CAD build for the part. Positions are in the model's coordinates, mm. Face numbers are marked on the shaded views. Round coordinates to 2 decimals unless told otherwise and drop trailing zeros. Loops run counter-clockwise (first coordinate to the right, second up) from the corner with the lowest first, then second, coordinate; pieces in that order, holes last.
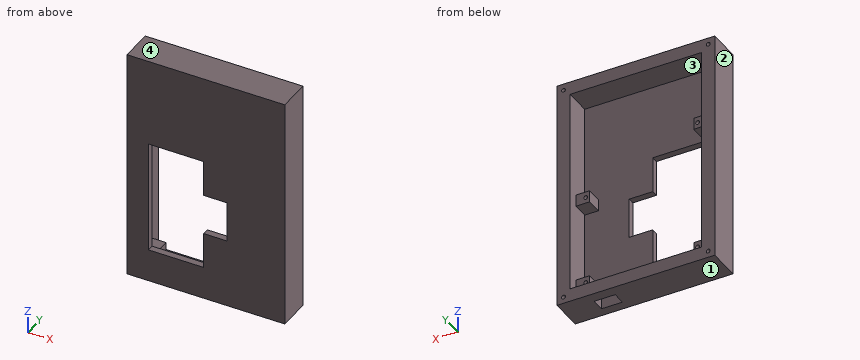
Autodesk Inventor part; units mm, degrees
ref_plane "YZ Plane" through (0, 0, 0) normal (1, 0, 0) x (0, 1, 0)
ref_plane "XZ Plane" through (0, 0, 0) normal (0, 1, 0) x (-1, 0, 0)
ref_plane "XY Plane" through (0, 0, 0) normal (0, 0, 1) x (1, 0, 0)
sketch "Sketch1" plane through (0, 0, 0) normal (0, 1, 0) x (-1, 0, 0)
  line L0 (3.609, 163.5234) -> (-116.891, 163.5234)
  line L1 (-116.891, 163.5234) -> (-116.891, -14.4766)
  line L2 (-116.891, -14.4766) -> (3.609, -14.4766)
  line L3 (3.609, -14.4766) -> (3.609, 163.5234)
  dimension "d1" = 178
  dimension "d2" = 120.5
extrude "Extrusion1" add sketch "Sketch1" along normal blind 25
sketch "Sketch2" plane through (0, 25, 0) normal (0, 1, 0) x (1, 0, 0)
  line L0 (6.391, -153.5234) -> (106.891, -153.5234)
  line L1 (106.891, -153.5234) -> (106.891, 4.4766)
  line L2 (106.891, 4.4766) -> (6.391, 4.4766)
  line L3 (6.391, 4.4766) -> (6.391, -153.5234)
  line L4 (-3.609, -163.5234) -> (116.891, -163.5234)
  line L5 (116.891, -163.5234) -> (116.891, 14.4766)
  point P0 (0, 0)
  dimension "d5" = 158
  dimension "d6" = 100.5
  dimension "d7" = 10
  dimension "d8" = 10
extrude "Extrusion2" cut sketch "Sketch2" against normal blind 20
sketch "Sketch3" plane through (0, 5, 0) normal (0, 1, 0) x (1, 0, 0)
  line L0 (12.891, -96.5234) -> (54.891, -96.5234)
  line L1 (54.891, -96.5234) -> (54.891, -10.5234)
  line L2 (54.891, -10.5234) -> (12.891, -10.5234)
  line L3 (12.891, -10.5234) -> (12.891, -96.5234)
  line L4 (106.891, -153.5234) -> (6.391, -153.5234)
  line L5 (6.391, 4.4766) -> (106.891, 4.4766)
  line L6 (6.391, -153.5234) -> (6.391, 4.4766)
  line L7 (54.891, -69.0234) -> (72.891, -69.0234)
  line L8 (72.891, -69.0234) -> (72.891, -38.0234)
  line L9 (72.891, -38.0234) -> (54.891, -38.0234)
  line L10 (54.891, -38.0234) -> (54.891, -69.0234)
  line L11 (106.891, 4.4766) -> (106.891, -153.5234)
  line L12 (12.891, -55.0234) -> (106.891, -55.0234)
  point P0 (0, 0)
  dimension "d11" = 57
  dimension "d12" = 15
  dimension "d13" = 6.5
  dimension "d14" = 0
  dimension "d15" = 42
  dimension "d16" = 34
  dimension "d17" = 42.5
  dimension "d18" = 84.5
  dimension "d19" = 41.5
  dimension "d20" = 44.5
  dimension "d21" = 14
extrude "Extrusion3" cut sketch "Sketch3" against normal through all contours L3 L12 L1 L0 | L3 L2 L1 L12 | L1 L12 L8 L7 | L1 L9 L8 L12
sketch "Sketch4" plane through (0, 5, 0) normal (0, 1, 0) x (1, 0, 0)
  line L0 (6.391, -7.5234) -> (16.891, -7.5234)
  line L1 (16.891, -7.5234) -> (16.891, 1.4766)
  line L2 (16.891, 1.4766) -> (6.391, 1.4766)
  line L3 (6.391, 1.4766) -> (6.391, -7.5234)
  line L4 (6.391, -153.5234) -> (6.391, 4.4766)
  line L5 (6.391, 4.4766) -> (106.891, 4.4766)
  line L6 (6.391, -153.5234) -> (6.391, 4.4766)
  line L7 (6.391, -53.5234) -> (106.891, -53.5234)
  line L8 (12.891, -10.5234) -> (54.891, -10.5234)
  line L9 (6.391, -99.5234) -> (16.891, -99.5234)
  line L10 (16.891, -99.5234) -> (16.891, -108.5234)
  line L11 (16.891, -108.5234) -> (6.391, -108.5234)
  line L12 (6.391, -108.5234) -> (6.391, -99.5234)
  line L13 (106.891, -153.5234) -> (6.391, -153.5234)
  line L14 (56.641, -153.5234) -> (56.641, 4.4766)
  line L15 (6.391, 4.4766) -> (106.891, 4.4766)
  line L16 (-3.609, 14.4766) -> (-3.609, -163.5234)
  line L17 (106.891, -7.5234) -> (96.391, -7.5234)
  line L18 (96.391, -7.5234) -> (96.391, 1.4766)
  line L19 (96.391, 1.4766) -> (106.891, 1.4766)
  line L20 (106.891, 1.4766) -> (106.891, -7.5234)
  line L21 (108.391, -37.5234) -> (6.391, -37.5234)
  line L22 (106.891, -67.5234) -> (96.391, -67.5234)
  line L23 (106.891, -76.5234) -> (106.891, -67.5234)
  line L24 (96.391, -67.5234) -> (96.391, -76.5234)
  line L25 (96.391, -76.5234) -> (106.891, -76.5234)
  line L26 (54.891, -96.5234) -> (12.891, -96.5234)
  point P0 (0, 0)
  dimension "d24" = 0
  dimension "d25" = 10.5
  dimension "d26" = 9
  dimension "d27" = 3
  dimension "d28" = 43
  dimension "d29" = 60.25
  dimension "d30" = 30
  dimension "d37" = 43
extrude "Extrusion4" add sketch "Sketch4" along normal blind 12 contours L3 L2 L1 L0 | L9 L10 L11 L4 | L17 L18 L19 L20 | L23 L25 L24 L22
sketch "Sketch6" plane through (0, 17, 0) normal (0, 1, 0) x (1, 0, 0)
  circle A0 centre (13.891, -3.0234) radius 1.5
  line L0 (6.391, -153.5234) -> (6.391, 4.4766)
  line L1 (16.891, 1.4766) -> (6.391, 1.4766)
  line L2 (6.391, -53.5234) -> (108.8142, -53.5234)
  line L3 (12.891, -10.5234) -> (54.891, -10.5234)
  line L4 (6.391, -108.5234) -> (16.891, -108.5234)
  circle A1 centre (13.891, -104.0234) radius 1.5
  line L5 (56.641, -153.5234) -> (56.641, 4.4766)
  line L6 (-3.609, 14.4766) -> (-3.609, -163.5234)
  circle A2 centre (99.391, -3.0234) radius 1.5
  line L7 (106.891, -7.5234) -> (106.891, -67.5234)
  line L8 (106.891, -37.5234) -> (6.391, -37.5234)
  line L9 (96.391, -7.5234) -> (106.891, -7.5234)
  circle A3 centre (99.391, -72.0234) radius 1.5
  line L10 (106.891, 4.4766) -> (106.891, -153.5234)
  line L11 (106.891, 1.4766) -> (96.391, 1.4766)
  point P0 (0, 0)
  dimension "d33" = 3
  dimension "d34" = 7.5
  dimension "d35" = 4.5
  dimension "d36" = 43
  dimension "d38" = 110
  dimension "d39" = 4.5
  dimension "d40" = 7.5
  dimension "d41" = 60.25
  dimension "d42" = 30
  dimension "d43" = 69
  dimension "d44" = 7.5
  dimension "d45" = 7.5
  dimension "d46" = 4.5
hole "Hole1" at (13.891, 17, 3.0234) at (13.891, 17, 104.0234) at (99.391, 17, 72.0234) at (99.391, 17, 3.0234) direction (0, -1, 0) diameter 3 depth 10 tip angle 118
thread "Thread1"
thread "Thread2"
thread "Thread3"
thread "Thread4"
sketch "Sketch7" plane through (0, 25, 0) normal (0, 1, 0) x (1, 0, 0)
  circle A0 centre (1.391, -158.5234) radius 1.5
  line L0 (-3.609, -163.5234) -> (116.891, -163.5234)
  line L1 (-3.609, 14.4766) -> (-3.609, -163.5234)
  line L2 (-3.609, 14.4766) -> (-3.609, -163.5234)
  line L3 (-3.609, -74.5234) -> (116.891, -74.5234)
  line L4 (116.891, -163.5234) -> (116.891, 14.4766)
  circle A1 centre (1.391, 9.4766) radius 1.5
  line L5 (56.641, -163.5234) -> (56.641, 14.4766)
  line L6 (116.891, 14.4766) -> (-3.609, 14.4766)
  circle A2 centre (111.891, -158.5234) radius 1.5
  circle A3 centre (111.891, 9.4766) radius 1.5
  point P0 (0, 0)
  dimension "d62" = 3
  dimension "d63" = 5
  dimension "d64" = 5
  dimension "d65" = 89
  dimension "d66" = 60.25
hole "Hole2" at (1.391, 25, 158.5234) at (1.391, 25, -9.4766) at (111.891, 25, -9.4766) at (111.891, 25, 158.5234) direction (0, -1, 0) diameter 3 depth 20 tip angle 118
thread "Thread5"
thread "Thread6"
thread "Thread7"
thread "Thread8"
sketch "Sketch8" plane through (6.391, 25, -4.4766) normal (0, 0, 1) x (1, 0, 0)
  line L0 (70.5, -18) -> (86.5, -18)
  line L1 (86.5, -18) -> (86.5, -8)
  line L2 (86.5, -8) -> (70.5, -8)
  line L3 (70.5, -8) -> (70.5, -18)
  line L4 (100.5, 0) -> (100.5, -20)
  line L5 (0, 0) -> (100.5, 0)
  line L6 (0, -20) -> (100.5, -20)
  point P0 (-6.391, -25)
  dimension "d82" = 14
  dimension "d83" = 16
  dimension "d84" = 8
  dimension "d85" = 2
extrude "Extrusion5" cut sketch "Sketch8" against normal through all
properties part number "cabin_front"
Item 1: Cut at C-C, the plane y = 22. Give the cut face in (x, z).
Answers follow:
outline: (-3.61, -14.48) - (116.89, -14.48) - (116.89, 163.52) - (-3.61, 163.52) - close; hole circle Ø3 at (1.39, -9.48); hole circle Ø3 at (1.39, 158.52); hole (6.39, -4.48) - (106.89, -4.48) - (106.89, 153.52) - (6.39, 153.52) - close; hole circle Ø3 at (111.89, -9.48); hole circle Ø3 at (111.89, 158.52)
Item 2: Cut at A-A, the plane z = 53.5. Give the cut face in (x, y), plus the area to 4 significant figures.
Answers follow:
outline: (-3.61, 0) - (12.89, 0) - (12.89, 5) - (6.39, 5) - (6.39, 25) - (-3.61, 25) - close; (72.89, 0) - (116.89, 0) - (116.89, 25) - (106.89, 25) - (106.89, 5) - (72.89, 5) - close
area: 702.5 mm2
Item 3: Flat gauge pins, fed straight in: P1, Ø4.5, axis at x = 100, z = 74, coming from the +Y side; P2, Ø2.5, axis at x = 99.39, z = 72.02, coming from the +Y side. Where does each tip first touch, or does it go through?
Answers follow:
P1: stops at y = 17
P2: stops at y = 6.85
Item 4: Cut at B-B, the plane x = 81. Give the cut face in (y, z), plus the area to 3 significant figures.
Answers follow:
outline: (0, -14.48) - (7, -14.48) - (7, -4.48) - (5, -4.48) - (5, 153.52) - (25, 153.52) - (25, 163.52) - (0, 163.52) - close; (17, -14.48) - (25, -14.48) - (25, -4.48) - (17, -4.48) - close
area: 1,190 mm2
Item 5: Two-plate mould, pull along Z, no slides. Class the marked faces 1, 2, 3 and 4: released by +Z, released by -Z, zero draft, split by the parting line, or undercut.
Answers follow:
face 1: released by -Z
face 2: zero draft
face 3: undercut
face 4: released by +Z
Item 6: Cut at D-D, the plane z = 136. Give the cut face in (x, y), plus the area to 3 significant figures.
Answers follow:
outline: (-3.61, 0) - (116.89, 0) - (116.89, 25) - (106.89, 25) - (106.89, 5) - (6.39, 5) - (6.39, 25) - (-3.61, 25) - close
area: 1,000 mm2
Item 7: Probe line 1 (Z direction, x = 26, y = 9.5); line 2 (X direction, y = 9.75, z = 117); line 3 (Z direction, x = 60, y = 3.25). List the from-to ranges inside material, lowest first.
Answers follow:
line 1: z = -14.48 to -4.48, 153.52 to 163.52
line 2: x = -3.61 to 6.39, 106.89 to 116.89
line 3: z = -14.48 to 38.02, 69.02 to 163.52
